Part model, mm, in its own coordinate system. Face numbers are marked on the shaded views. Give positions to 0.01 mm unless a question says otherwise; leave off trailing zeros. Write each loop counter-clockwise with the first axis right and the second up, starting at its lowest first coordinate (ties: lowest second). Pieces come first, ordered by that corner, then holes. Notation, with made-up numbers: M -26,-8.75 L -14,-8.75 A7 ccw -14,4.25 Z; hole C 77.25,-2.5 d10. An arc over 180 degrees is marked long. Use a Markdown table: item, result.
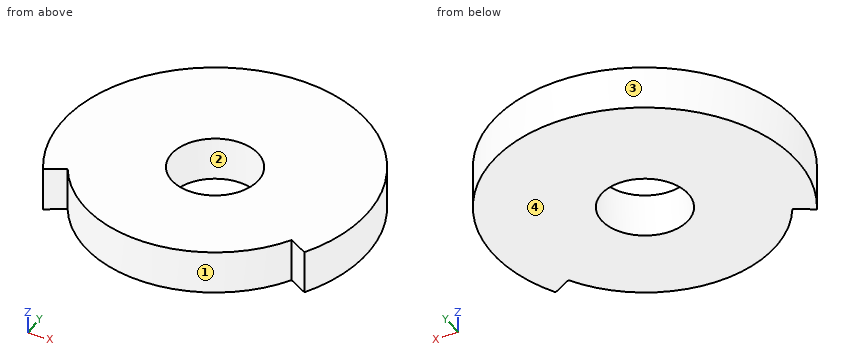
```python
from build123d import *

# Parameters (mm, degrees)
SKETCH1_R           = 1
BOSS_EXTRUDE1_DEPTH = 1


with BuildPart() as part:
    # Sketch1 → Boss-Extrude1 (new body)
    with BuildSketch(Plane(origin=(0, 0, 0), x_dir=(-1, 0, 0), z_dir=(0, 0, -1))):
        with BuildLine():
            Line((-3.031088913, -1.75), (-2.598076211, -1.5))
            ThreePointArc((-2.598076211, -1.5), (0, -3), (2.598076211, -1.5))
            Line((2.598076211, -1.5), (3.031088913, -1.75))
            ThreePointArc((3.031088913, -1.75), (0, 3.5), (-3.031088913, -1.75))
        make_face()
        with Locations(Location((0, 0, 0), (0, 0, 180))):
            Circle(SKETCH1_R, mode=Mode.SUBTRACT)
    extrude(amount=-BOSS_EXTRUDE1_DEPTH)


solid = part.part
```
1. Cut at A-A, the plane x = 0. Give the cut face in (y, z), then the cut area to 3 significant figures.
Findings below:
| item | result |
|---|---|
| outline | M -3,0 L -1,0 L -1,1 L -3,1 Z; M 1,0 L 3.5,0 L 3.5,1 L 1,1 Z |
| area | 4.50 mm2 |
2. Cut at B-B, the plane z = 0.85. Give the cut face in (x, y).
Findings below:
| item | result |
|---|---|
| outline | M -3.03,-1.75 L -2.6,-1.5 A3 ccw 2.6,-1.5 L 3.03,-1.75 A3.5 ccw long Z; hole C 0,0 d2 |
3. Drop a flat-ended pin along its axis: P1, Ø1.8, axis at x = 0, y = 0, coming from the +Z side. Give the stop position or say it passes through.
Findings below:
| item | result |
|---|---|
| P1 | through |
4. Cut at D-D, the plane x = 1.25. Give the cut face in (y, z), then the cut area to 3 significant figures.
Findings below:
| item | result |
|---|---|
| outline | M -2.73,0 L 3.27,0 L 3.27,1 L -2.73,1 Z |
| area | 6.00 mm2 |
5. Drill centre lines: L1, parallel to Y at x = 0, z = 0.45; L2, parallel to X at y = 0.5, z = 0.8; L3, parallel to X at y = 1.75, z = 0.5. Where is each one in solid material? Low to high.
Findings below:
| item | result |
|---|---|
| L1 | -3 to -1, 1 to 3.5 |
| L2 | -3.46 to -0.87, 0.87 to 3.46 |
| L3 | -3.03 to 3.03 |
6. Two-plate mould, pull along Y, no slides. Class the marked faces 1, 2, 3 and 4: released by +Y, released by -Y, zero draft, split by the parting line, or undercut.
Findings below:
| item | result |
|---|---|
| face 1 | released by -Y |
| face 2 | undercut |
| face 3 | split by the parting line |
| face 4 | zero draft |
7. Cut at C-C, the plane y = 0.25. Give the cut face in (x, z).
Findings below:
| item | result |
|---|---|
| outline | M -3.49,0 L -0.97,0 L -0.97,1 L -3.49,1 Z; M 0.97,0 L 3.49,0 L 3.49,1 L 0.97,1 Z |
